Geometry: see drawing. Coordinates: mm, zero at the bounding-box minimum. Coordinates: 2 decimals unless noted, no trailing zeros. Write each loop counter-clockwise with the first axis right and the second up, starting at its lowest first coordinate (ties: lowest second). Pieces come first, ordered by that corner, then holes. Notation, with made-up numbers: (37.5, -16.5) - (47.5, -16.5) arc R17 cw to (47.5, -4.5) - close; hole circle Ø5 at (76.5, 30.25). An arc over 180 degrees is marked (long way). One line per question, with ' | ' between items. Start each with the question number.
Q1. Cut plane B-B, the plane x = 53.87. Return loops of the section in (y, z) (3 decimals), plus the area to 3 significant figures.
Q2. Cut plane D-D, the plane y = 0.7. Give the number of separate pieces and of enclosed holes in the cut face, plus the area to 3 significant figures.
Q3. Cut plane A-A, the plane z = 41. Return loops of the section in (x, y) (3 decimals), plus the area to 3 significant figures.
Q4. Cut plane C-C, the plane z = 8. Return loops of the section in (x, y), plus the area to 3 significant figures.
Q5. Line query: line 1 (X direction, y = 0.9, z = 41) (3 decimals); line 2 (X direction, y = 1.15, z = 39); line 3 (X direction, y = 0.9, z = 8). Output: solid intervals per line, ascending.
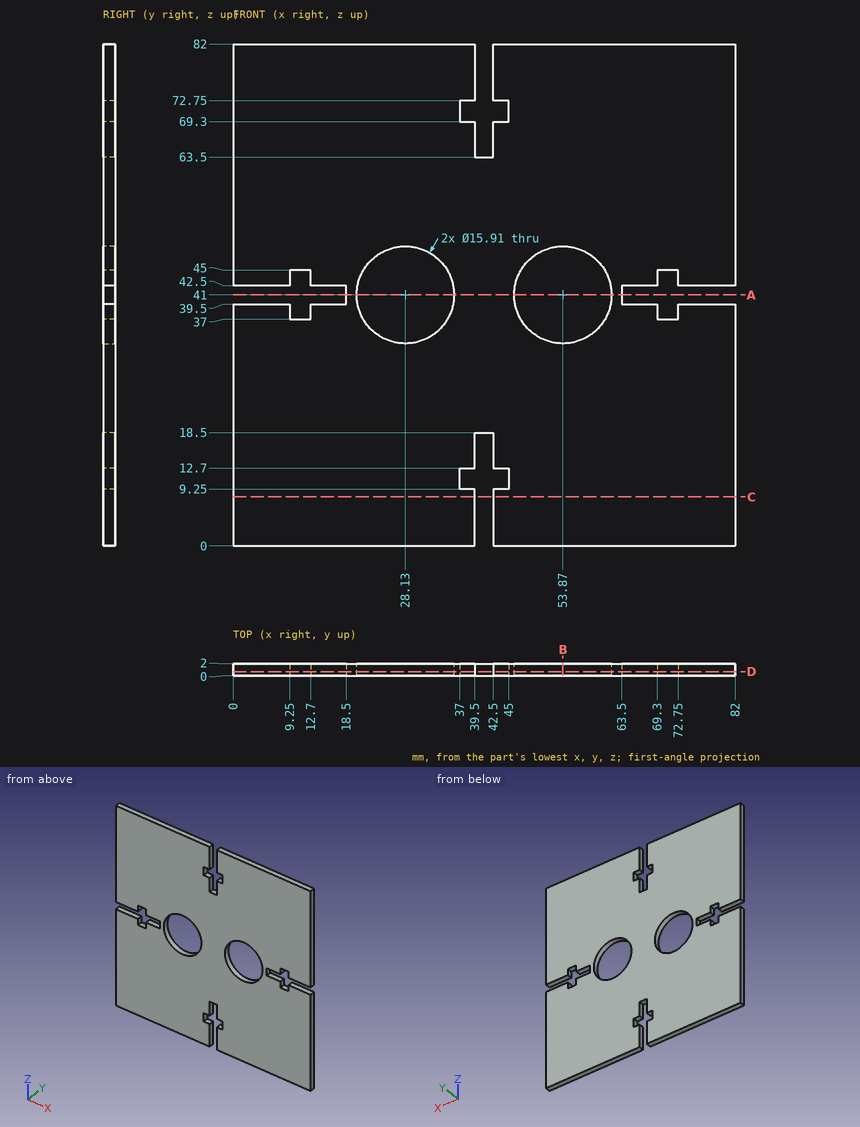
Reply:
1) outline: (0, 0) - (2, 0) - (2, 33.045) - (0, 33.045) - close; (0, 48.955) - (2, 48.955) - (2, 82) - (0, 82) - close | area: 132 mm^2
2) separate pieces: 1 | enclosed holes: 2 | area: 6,040 mm^2
3) outline: (18.5, 0) - (20.175, 0) - (20.175, 2) - (18.5, 2) - close; (36.085, 0) - (45.915, 0) - (45.915, 2) - (36.085, 2) - close; (61.825, 0) - (63.5, 0) - (63.5, 2) - (61.825, 2) - close | area: 26.4 mm^2
4) outline: (0, 0) - (39.5, 0) - (39.5, 2) - (0, 2) - close; (42.5, 0) - (82, 0) - (82, 2) - (42.5, 2) - close | area: 158 mm^2
5) line 1: x = 18.5 to 20.175, 36.085 to 45.915, 61.825 to 63.5 | line 2: x = 0 to 9.25, 12.7 to 20.43, 35.83 to 46.17, 61.57 to 69.3, 72.75 to 82 | line 3: x = 0 to 39.5, 42.5 to 82
